Geometry: final body of the model. Coordinates: model frame, mm. A direction names the side the tool comes from. Round coordinates to 2 decimals unless told otherwise and drop trailing zeros. Loops run counter-clockwise (first coordinate to the right, second up) from the corner with the lowest first, then second, coordinate; pieces in that order, holes last. Notation, with made-up numbers: (55.25, -22.5) - (64.25, -22.5) arc R6 cw to (64.25, -13.5) - close; hole circle Ø9 at (-28.75, 3). An arc over 180 degrees is marked (long way). Answer as CSV lines item,"result".
from build123d import *

# Parameters (mm, degrees)
F1_DEPTH = 12.7508
F2_R     = 1.27


with BuildPart() as f1:
    # F0 (on Top) → F1 (new body)
    with BuildSketch(Plane.XY):
        with BuildLine():
            Line((-5.912621, -12.42536), (-3.132528, -7.610098))
            ThreePointArc((-3.132528, -7.610098), (0, -8.2296), (3.132528, -7.610098))
            Line((3.132528, -7.610098), (5.912621, -12.42536))
            ThreePointArc((5.912621, -12.42536), (8.73125, -15.122969), (7.804367, -11.33316))
            Line((7.804367, -11.33316), (5.024274, -6.517898))
            ThreePointArc((5.024274, -6.517898), (7.127043, -4.1148), (8.156802, -1.0922))
            Line((8.156802, -1.0922), (13.716988, -1.0922))
            ThreePointArc((13.716988, -1.0922), (15.999344, -1.950754), (17.4625, 0))
            ThreePointArc((17.4625, 0), (15.999344, 1.950754), (13.716988, 1.0922))
            Line((13.716988, 1.0922), (8.156802, 1.0922))
            ThreePointArc((8.156802, 1.0922), (7.127043, 4.1148), (5.024274, 6.517898))
            Line((5.024274, 6.517898), (7.804367, 11.33316))
            ThreePointArc((7.804367, 11.33316), (8.73125, 15.122969), (5.912621, 12.42536))
            Line((5.912621, 12.42536), (3.132528, 7.610098))
            ThreePointArc((3.132528, 7.610098), (0, 8.2296), (-3.132528, 7.610098))
            Line((-3.132528, 7.610098), (-5.912621, 12.42536))
            ThreePointArc((-5.912621, 12.42536), (-8.73125, 15.122969), (-7.804367, 11.33316))
            Line((-7.804367, 11.33316), (-5.024274, 6.517898))
            ThreePointArc((-5.024274, 6.517898), (-7.127043, 4.1148), (-8.156802, 1.0922))
            Line((-8.156802, 1.0922), (-13.716988, 1.0922))
            ThreePointArc((-13.716988, 1.0922), (-17.4625, 0), (-13.716988, -1.0922))
            Line((-13.716988, -1.0922), (-8.156802, -1.0922))
            ThreePointArc((-8.156802, -1.0922), (-7.127043, -4.1148), (-5.024274, -6.517898))
            Line((-5.024274, -6.517898), (-7.804367, -11.33316))
            ThreePointArc((-7.804367, -11.33316), (-8.73125, -15.122969), (-5.912621, -12.42536))
        make_face()
        with BuildLine():
            ThreePointArc((-5.193253, 2.355069), (-3.351728, 4.613258), (-0.635, 5.666833))
            Line((-0.635, 5.666833), (-0.635, 6.6548))
            Line((-0.635, 6.6548), (0.635, 6.6548))
            Line((0.635, 6.6548), (0.635, 5.666833))
            ThreePointArc((0.635, 5.666833), (3.351728, 4.613258), (5.193253, 2.355069))
            Line((5.193253, 2.355069), (6.132865, 2.660367))
            Line((6.132865, 2.660367), (6.525317, 1.452525))
            Line((6.525317, 1.452525), (5.585705, 1.147227))
            ThreePointArc((5.585705, 1.147227), (5.42321, -1.762108), (3.844607, -4.211321))
            Line((3.844607, -4.211321), (4.425319, -5.010603))
            Line((4.425319, -5.010603), (3.397868, -5.75709))
            Line((3.397868, -5.75709), (2.817155, -4.957808))
            ThreePointArc((2.817155, -4.957808), (0, -5.7023), (-2.817155, -4.957808))
            Line((-2.817155, -4.957808), (-3.397868, -5.75709))
            Line((-3.397868, -5.75709), (-4.425319, -5.010603))
            Line((-4.425319, -5.010603), (-3.844607, -4.211321))
            ThreePointArc((-3.844607, -4.211321), (-5.42321, -1.762108), (-5.585705, 1.147227))
            Line((-5.585705, 1.147227), (-6.525317, 1.452525))
            Line((-6.525317, 1.452525), (-6.132865, 2.660367))
            Line((-6.132865, 2.660367), (-5.193253, 2.355069))
        make_face(mode=Mode.SUBTRACT)
    extrude(amount=F1_DEPTH)

    # F2
    f2_edges = [f1.edges().sort_by_distance(p)[0] for p in [
        (-3.132528, 7.610098, 6.3754),
        (5.024274, 6.517898, 6.3754),
        (8.156802, 1.0922, 6.3754),
        (3.132528, 7.610098, 6.3754),
        (-5.024274, 6.517898, 6.3754),
        (-8.156802, 1.0922, 6.3754),
        (-5.024274, -6.517898, 6.3754),
        (-8.156802, -1.0922, 6.3754),
        (-3.132528, -7.610098, 6.3754),
        (3.132528, -7.610098, 6.3754),
        (5.024274, -6.517898, 6.3754),
        (8.156802, -1.0922, 6.3754),
    ]]
    fillet(f2_edges, radius=F2_R)


solid = f1.part
(1) Pin query (flat end, axial travel): P1, Ø1.1, axis at y = 6, z = 7, coming from the +X side; P2, Ø2, axis at x = 6, z = 1.5, coming from the +Y side; P3, Ø3, axis at x = 1, z = 2.5, coming from the +Y side. Return the tip coordinate at first contact, or that it passes through.
Findings below:
P1,"x = 6.17"
P2,"y = 15.27"
P3,"y = 8.23"
(2) Material intervals for line 1 along Y through (x, z) = (-9.5, 3.25); line 2 along Y through (x, z) = (7, 1.75); line 3 along X through (y, z) = (14, 8), sorted ascending.
Findings below:
line 1,"-14.33 to -12.39, -1.09 to 1.09, 12.39 to 14.33"
line 2,"-15.27 to -9.94, -4.33 to 4.33, 9.94 to 15.27"
line 3,"-9.64 to -5.79, 5.79 to 9.64"
(3) Section C-C (x = 10.5). Output: boundary loops of the cut face in (y, z).
Findings below:
outline,"(-1.09, 0) - (1.09, 0) - (1.09, 12.75) - (-1.09, 12.75) - close"
(4) Access query for faces 5 (the face through (0.041, -5.702, 6.286)), 6 (the face through (-7.14, -4.09, 6.29)), 7 (the face through (3.024, 7.969, 6.465)). Directions: +Z, -Z, +X, -X, +Y, -Y. A direction counts if a zero-diameter tool reaches every point of the face in a straight line with its end or side. Return the directions, or none.
Findings below:
face 5,"+Z, -Z"
face 6,"+Z, -Z, -X"
face 7,"+Z, -Z, +Y"
(5) Section D-D (x = -15). Output: boundary loops of the cut face in (y, z).
Findings below:
outline,"(-1.99, 0) - (1.99, 0) - (1.99, 12.75) - (-1.99, 12.75) - close"
(6) Section B-B (y = 13). Output: boundary loops of the cut face in (x, z).
Findings below:
outline,"(-9.71, 0) - (-5.72, 0) - (-5.72, 12.75) - (-9.71, 12.75) - close; (5.72, 0) - (9.71, 0) - (9.71, 12.75) - (5.72, 12.75) - close"
(7) Section A-A (x = 0). Output: boundary loops of the cut face in (y, z), and give its area (3 significant figures).
Findings below:
outline,"(-8.23, 0) - (-5.7, 0) - (-5.7, 12.75) - (-8.23, 12.75) - close; (6.65, 0) - (8.23, 0) - (8.23, 12.75) - (6.65, 12.75) - close"
area,"52.3 mm2"
(8) Draft query along X for faces 1 (the face through (7.111, -4.142, 6.286)), 2 (the face through (-3.9, -5.39, 6.29)), 3 (the face through (1, 6, 12.751)), 4 (the face through (-7.111, 4.142, 6.286)). Return one class per face: pulls with the +X half, pulls with the -X half, needs draft (parallel to the pull), parting line crosses it, or undercut.
Findings below:
face 1,"pulls with the +X half"
face 2,"undercut"
face 3,"needs draft"
face 4,"pulls with the -X half"
